Answer from the drawing. Dimensions are ordinates in mm from the lowest x, y and z of the part. Give positions to 0.01 mm unless a question says otherwise; leave off trailing zeros. Order: outer loops, then holes, each group sorted by start corner. A loop starts at its lowest first (then second) coordinate and runs counter-clockwise, first axis right, second up. Notation, with made-up numbers: (62.25, 74.25) - (83.25, 74.25) arc R22 cw to (83.25, 87.25) - close; hole circle Ø5 at (39.5, 71.5). An arc over 180 degrees is marked (long way). Answer in a Markdown table with one row per item.
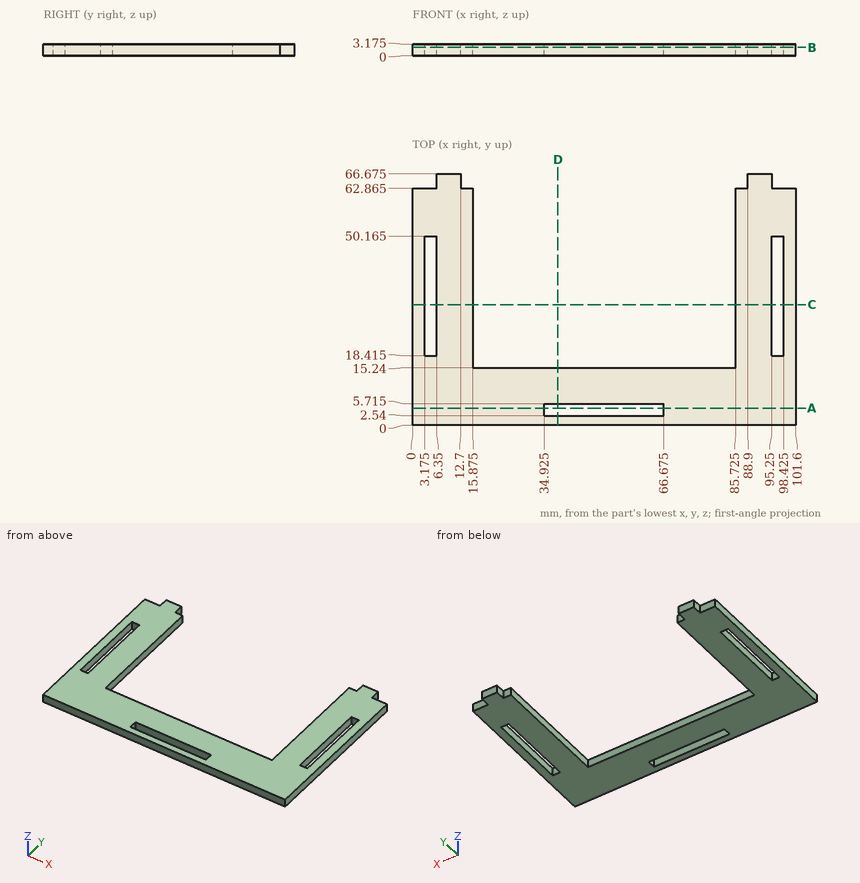
Item 1: Find section B-B on z = 2.25. Write down the section's boundary in (x, y) (3 decimals), then the cut area to 3 significant figures.
Answer block:
| item | result |
|---|---|
| outline | (0, 0) - (101.6, 0) - (101.6, 62.865) - (95.25, 62.865) - (95.25, 66.675) - (88.9, 66.675) - (88.9, 62.865) - (85.725, 62.865) - (85.725, 15.24) - (15.875, 15.24) - (15.875, 62.865) - (12.7, 62.865) - (12.7, 66.675) - (6.35, 66.675) - (6.35, 62.865) - (0, 62.865) - close; hole (3.175, 18.415) - (6.35, 18.415) - (6.35, 50.165) - (3.175, 50.165) - close; hole (34.925, 2.54) - (66.675, 2.54) - (66.675, 5.715) - (34.925, 5.715) - close; hole (95.25, 18.415) - (98.425, 18.415) - (98.425, 50.165) - (95.25, 50.165) - close |
| area | 2,810 mm² |
Item 2: Find section D-D on x = 38.5. Write down the section's boundary in (y, z) (3 decimals).
Answer block:
| item | result |
|---|---|
| outline | (0, 0) - (2.54, 0) - (2.54, 3.175) - (0, 3.175) - close; (5.715, 0) - (15.24, 0) - (15.24, 3.175) - (5.715, 3.175) - close |
Item 3: Find section C-C on y = 32. Write down the section's boundary in (x, z) (3 decimals), then the cut area to 3 significant figures.
Answer block:
| item | result |
|---|---|
| outline | (0, 0) - (3.175, 0) - (3.175, 3.175) - (0, 3.175) - close; (6.35, 0) - (15.875, 0) - (15.875, 3.175) - (6.35, 3.175) - close; (85.725, 0) - (95.25, 0) - (95.25, 3.175) - (85.725, 3.175) - close; (98.425, 0) - (101.6, 0) - (101.6, 3.175) - (98.425, 3.175) - close |
| area | 80.6 mm² |
Item 4: Each of these flat-tipped pins is pushed along its axis until it touches: P1, Ø6, axis at x = 63.5, y = 18.5, coming from the -Z side; P2, Ø1, axis at y = 64.5, z = 2.5, coming from the -X side; P3, Ø1.6, axis at y = 64.5, z = 1.5, coming from the +X side. Where does it stop, or does it pass through?
Answer block:
| item | result |
|---|---|
| P1 | through |
| P2 | x = 6.35 |
| P3 | x = 95.25 |
Item 5: Consider line 1 (X direction, y = 38, z = 0.9) (3 decimals); line 2 (Y direction, x = 64, z = 0.7) (3 decimals); line 3 (X direction, y = 5, z = 2.6) (3 decimals). Determine where each line is inside the solid, lowest interval first.
Answer block:
| item | result |
|---|---|
| line 1 | 0 to 3.175, 6.35 to 15.875, 85.725 to 95.25, 98.425 to 101.6 |
| line 2 | 0 to 2.54, 5.715 to 15.24 |
| line 3 | 0 to 34.925, 66.675 to 101.6 |
Item 6: Find section A-A on y = 4.5. Write down the section's boundary in (x, z) (3 decimals), then the cut area to 3 significant figures.
Answer block:
| item | result |
|---|---|
| outline | (0, 0) - (34.925, 0) - (34.925, 3.175) - (0, 3.175) - close; (66.675, 0) - (101.6, 0) - (101.6, 3.175) - (66.675, 3.175) - close |
| area | 222 mm² |
